from build123d import *

# Parameters (mm, degrees)
SKETCH1_W           = 80
SKETCH1_H           = 50
BOSS_EXTRUDE1_DEPTH = 5
SKETCH2_R           = 1.5
CUT_EXTRUDE1_DEPTH  = 5
FILLET2_R           = 10


with BuildPart() as part:
    # Sketch1 → Boss-Extrude1 (new body)
    with BuildSketch(Plane.XY):
        Rectangle(SKETCH1_W, SKETCH1_H)
    extrude(amount=BOSS_EXTRUDE1_DEPTH)

    # Sketch2 → Cut-Extrude1 (cut)
    with BuildSketch(Plane.XY.offset(5)):
        with Locations((-21.727182294, 13)):
            Circle(SKETCH2_R)
        with Locations((-8.727182294, 0)):
            Circle(SKETCH2_R)
        with Locations((-21.727182294, -13)):
            Circle(SKETCH2_R)
        with Locations((-34.727182294, 0)):
            Circle(SKETCH2_R)
    extrude(amount=-CUT_EXTRUDE1_DEPTH, mode=Mode.SUBTRACT)

    # Fillet2
    fillet2_edges = [part.edges().sort_by_distance(p)[0] for p in [
        (40, -25, 2.5),
        (-40, -25, 2.5),
        (-40, 25, 2.5),
        (40, 25, 2.5),
    ]]
    fillet(fillet2_edges, radius=FILLET2_R)


solid = part.part
The model under review builds one solid part; all positions refer to its coordinate system, in mm. Round coordinates to 2 decimals unless told otherwise and drop trailing zeros. Order: outer loops, then holes, each group sorted by start corner. A loop starts at its lowest first (then second) coordinate and runs counter-clockwise, first axis right, second up. Notation, with made-up numbers: (-24, 77.5) -> (31, 77.5) arc R33 cw to (31, 108.5) -> close; hole circle Ø5 at (-12, -38). An arc over 180 degrees is marked (long way). Return JSON: item names as keys, results as strings.
1. Insertion check: P1, Ø6, axis at x = 15.5, y = -17, coming from the -Z side. The pin has a flat end and moves straight along its axis. Give the tip position at first contact, or say it passes through.
Answer block:
{"P1": "stops at z = 0"}
2. The part is to be moulded in two halves that separate along Y. For faces 1 (the face through (-40, 0, 2)), 2 (the face through (-20.296, 13.451, 2.535)), 3 (the face through (36.99, 22.15, 2.54)), 4 (the face through (0, -25, 2)), say which applies: +Y half, -Y half, draft (parallel to the pull), parting line (faces both ways), or undercut.
Answer block:
{"face 1": "draft", "face 2": "undercut", "face 3": "+Y half", "face 4": "-Y half"}
3. Take a section at A-A (y = 0). Write out the cut boundary in (x, z), then the cut area to 3 significant figures.
Answer block:
{"outline": "(-40, 0) -> (-36.23, 0) -> (-36.23, 5) -> (-40, 5) -> close; (-33.23, 0) -> (-10.23, 0) -> (-10.23, 5) -> (-33.23, 5) -> close; (-7.23, 0) -> (40, 0) -> (40, 5) -> (-7.23, 5) -> close", "area": "370 mm²"}
4. For L1, parallel to Y at x = -36, z = 2.95; L2, parallel to X at y = -20.5, z = 1.3; L3, parallel to Y at x = 33, z = 4.65, list the stretches that pass through material, from the lowest coordinate up. Write a range as [from, to].
Answer block:
{"L1": "y = [-23, -0.79], [0.79, 23]", "L2": "x = [-38.35, 38.35]", "L3": "y = [-24.54, 24.54]"}
5. Take a section at B-B (y = -13). Write out the cut boundary in (x, z).
Answer block:
{"outline": "(-40, 0) -> (-23.23, 0) -> (-23.23, 5) -> (-40, 5) -> close; (-20.23, 0) -> (40, 0) -> (40, 5) -> (-20.23, 5) -> close"}
6. Take a section at D-D (y = -22). Write out the cut boundary in (x, z), then the cut area to 3 significant figures.
Answer block:
{"outline": "(-37.14, 0) -> (37.14, 0) -> (37.14, 5) -> (-37.14, 5) -> close", "area": "371 mm²"}
7. Take a section at C-C (z = 1). Write out the cut boundary in (x, y).
Answer block:
{"outline": "(-40, -15) arc R10 ccw to (-30, -25) -> (30, -25) arc R10 ccw to (40, -15) -> (40, 15) arc R10 ccw to (30, 25) -> (-30, 25) arc R10 ccw to (-40, 15) -> close; hole circle Ø3 at (-34.73, 0); hole circle Ø3 at (-21.73, -13); hole circle Ø3 at (-21.73, 13); hole circle Ø3 at (-8.73, 0)"}
